Build history of the part. All positions in model axes, mm. Give positions to 0.01 mm unless a question says otherwise; leave off trailing zeros. Loops run counter-clockwise (first coordinate to the right, second up) from the corner with the lowest first, then second, coordinate; pieces in that order, holes last. Notation, with made-up numbers: (1.25, -37) -> (36.25, -37) arc R21 ccw to (36.25, -20) -> close; hole circle Ø3 at (81, 19.25). An arc over 180 degrees is marked (long way). One line per question, with ' | ' between items. Start each with the question number.
(1) Mould opens along Y. For faces 1 (the face through (3, 0, 2)), 2 (the face through (0, 0, 0)), 3 (the face through (5, 0, 1)), 4 (the face through (2.875, 0.033, -0.064)) say: pulls with the +Y half, pulls with the -Y half, needs draft (parallel to the pull), parting line crosses it, or undercut.
(2) Drill centre lines: L1, parallel to Z at x = 5, y = 0.7; L2, parallel to Y at x = 3.75, z = 0.05; L3, parallel to Z at x = 1.7, y = 0.1. Where is each one in solid material? Low to high. Write a range as from..to.
(3) Flat gauge pin, fed straight in: pin 1 Ø1 at (x, z) = (1.5, -1.5) entering from -Y. Where does the tip first touch, or does it go through?
(4) Slice it at A-A, the plane x = 4.35. Write the cut outline in (y, z).
Autodesk Inventor part; units mm, degrees
ref_plane "Work Plane1" through (3, 0, 0) normal (0, 0, 1) x (1, 0, 0)
ref_plane "YZ Plane" through (0, 0, 0) normal (1, 0, 0) x (0, 1, 0)
ref_plane "XZ Plane" through (0, 0, 0) normal (0, 1, 0) x (-1, 0, 0)
sketch "Skizze1" plane through (0, 0, 0) normal (0, 0, 1) x (1, 0, 0)
  line L0 (0, 0) -> (2.8333, 0)
  line L1 (6, 1.1547) -> (6, 2)
  line L2 (6, 2) -> (0, 2)
  line L3 (6, 1.1547) -> (3.5, 1.1547)
  line L4 (3.5, 1.1547) -> (2.8333, 0)
  line L5 (0, -0.4) -> (0, 2.4)
  line L6 (0, 2) -> (0, 0)
  dimension "d0" = 2.5
  dimension "d1" = 60
  dimension "d2" = 4
  dimension "d3" = 2.3094
  dimension "d5" = 6
revolve "Körper" add sketch "Skizze1" angle 360 about axis through (0, 0, 0) along (1, 0, 0)
sketch "Skizze2" plane through (6, 0, 0) normal (1, 0, 0) x (0, 1, 0)
  circle A0 centre (0, 0) radius 1.1547
  line L0 (-0.5774, 1) -> (0.5774, 1)
  line L1 (0.5774, 1) -> (1.1547, 0)
  line L2 (1.1547, 0) -> (0.5774, -1)
  line L3 (0.5774, -1) -> (-0.5774, -1)
  line L4 (-0.5774, -1) -> (-1.1547, 0)
  line L5 (-1.1547, 0) -> (-0.5774, 1)
  point P0 (0, 0)
  point P1 (0, 0)
extrude "Loch" add sketch "Skizze2" against normal up to next contours L1 A0 | A0 L2 | L0 A0 | A0 L3 | L5 A0 | A0 L4
thread "Gewinde"
chamfer "Fase1" distance 0.4294 angle 45 1 edges at (6, -2, 0) measured on face at (4, 1.9935, -0.1609)
chamfer "Fase2" distance 0.4294 angle 45 1 edges at (0, -2, 0) measured on face at (1.8569, 1.9935, -0.1609)
ref_plane "Work Plane1" through (3, 0, 0) normal (0, 0, 1) x (1, 0, 0)
equation "\"d0\" = INTI"
equation "\"d2\" = NND"
equation "\"d3\" = 1.1547 * SW"
equation "\"d5\" = NLG"
equation "\"d8\" = NLG"
equation "\"d10\" = -0.5 * GD1 + 0.5 * NND"
equation "\"d11\" = FAWI"
equation "\"d34\" = -0.5 * GD1 + 0.5 * NND"
equation "\"d12\" = -0.5 * GD1 + 0.5 * NND"
equation "\"d13\" = FAWI"
equation "\"d35\" = -0.5 * GD1 + 0.5 * NND"
equation "\"NND\" = 4"
equation "\"NLG\" = 6"
equation "\"INTI\" = 2.5"
equation "\"FAWI\" = 45deg"
equation "\"SW\" = 2"
equation "\"GD1\" = THREADDIA - 1.2269 * PTC"
equation "\"SPD\" = 2.5"
equation "\"GUL\" = 0.61345 * PTC"
equation "\"TOA\" = 30deg"
equation "\"THREADDIA\" = 4"
equation "\"PTC\" = 0.7"
equation "\"FAWI1\" = 45deg"
equation "\"GAL\" = 0.61345 * PTC"
equation "\"E0\" = 1.155 * SW"
properties part number "DIN 913 - M4 x 6" material "Stahl, weich"
Final values:
1) face 1: parting line crosses it | face 2: needs draft | face 3: undercut | face 4: undercut
2) L1: -1.87..-0.79, 0.79..1.87 | L2: -2..-1.13, 1.13..2 | L3: -2..2
3) pin 1: y = -1.73
4) outline: circle Ø4 at (0, 0); hole (-1.15, 0) -> (-0.58, -1) -> (0.58, -1) -> (1.15, 0) -> (0.58, 1) -> (-0.58, 1) -> close
